Model file for the job. Use its own axes, mm. Face numbers are marked on the shaded views. A direction names the side the tool comes from. Give positions to 0.01 mm unless a question says otherwise; leave off trailing zeros. Write each loop counter-clockwise with the first axis right and the second up, starting at its lowest first coordinate (ties: lowest second). Pieces come first, ordered by that corner, then holes. Notation, with made-up numbers: M 74,46.5 L 90,46.5 A14 ccw 90,65.5 Z; hole C -18.75,63.5 d10. An arc over 180 degrees is marked long. Answer as a JSON object with one key per item and string values. Group by question number.
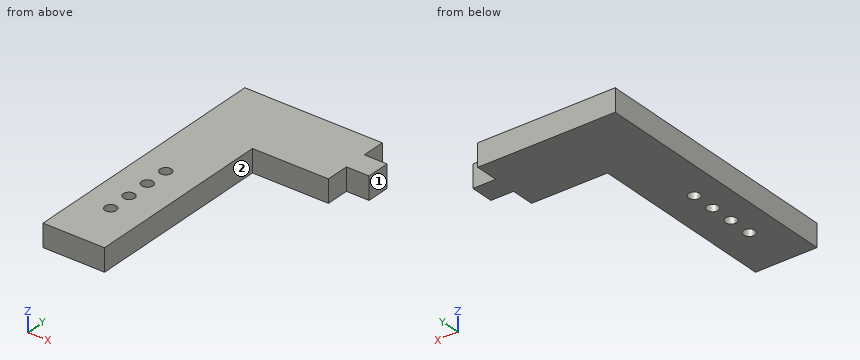
```python
from build123d import *

# Parameters (mm, degrees)
SKETCH1_W           = 13.462
SKETCH1_H           = 57.15
BOSS_EXTRUDE1_DEPTH = 4.9609375
SKETCH2_W           = 4.9609375
SKETCH2_H           = 15.24
BOSS_EXTRUDE2_DEPTH = 21.59
SKETCH5_R           = 1.2446
SKETCH5_R_2         = 1.25
SKETCH5_R_3         = 1.24968
CUT_EXTRUDE2_DEPTH  = 5.9609375
SKETCH6_OUTSIDE_W   = 20.407
SKETCH6_OUTSIDE_H   = 72.596
SKETCH6_OUTSIDE_W_2 = 4.9609375
SKETCH6_OUTSIDE_H_2 = 5.08
CUT_EXTRUDE3_DEPTH  = 4.9609375


with BuildPart() as part:
    # Sketch1 → Boss-Extrude1 (new body)
    with BuildSketch(Plane.XY):
        Rectangle(SKETCH1_W, SKETCH1_H)
    extrude(amount=BOSS_EXTRUDE1_DEPTH)

    # Sketch2 → Boss-Extrude2 (add)
    with BuildSketch(Plane(origin=(6.731, 0, 0), x_dir=(0, 0, -1), z_dir=(1, 0, 0))):
        with Locations((-2.48046875, 20.955)):
            Rectangle(SKETCH2_W, SKETCH2_H)
    extrude(amount=BOSS_EXTRUDE2_DEPTH)

    # Sketch5 → Cut-Extrude2 (cut, through all)
    with BuildSketch(Plane(origin=(0, 0, 0), x_dir=(-1, 0, 0), z_dir=(0, 0, -1))):
        with Locations((0.502153829, -17.4625)):
            Circle(SKETCH5_R)
        with Locations((0.502153829, -12.2625)):
            Circle(SKETCH5_R_2)
        with Locations((0.502153829, -7.0625)):
            Circle(SKETCH5_R_3)
        with Locations((0.502153829, -1.8625)):
            Circle(SKETCH5_R_3)
    extrude(amount=-CUT_EXTRUDE2_DEPTH, mode=Mode.SUBTRACT)

    # Sketch6 outside → Cut-Extrude3 (cut)
    with BuildSketch(Plane(origin=(28.321, 0, 0), x_dir=(0, 0, -1), z_dir=(1, 0, 0))):
        with Locations((-2.4805, 0)):
            Rectangle(SKETCH6_OUTSIDE_W, SKETCH6_OUTSIDE_H)
        with Locations((-2.48046875, 20.955)):
            Rectangle(SKETCH6_OUTSIDE_W_2, SKETCH6_OUTSIDE_H_2, mode=Mode.SUBTRACT)
    extrude(amount=-CUT_EXTRUDE3_DEPTH, mode=Mode.SUBTRACT)


solid = part.part
```
Q1. Drop flat-ended pins along their axis: P1, Ø1.5, axis at x = 25, z = 1.5, coming from the +Y side (3 decimals); P2, Ø2.5, axis at y = 15, z = 3, coming from the +X side; P3, Ø2.5, axis at y = -14, z = 3.5, coming from the +X side. Give the stop position or say it passes through.
Q2. Slice it at B-B, the plane x = 26.5. Write the cut outline in (y, z) (3 decimals).
Q3. Wall check: L1, parallel to Y at x = -1, z = 0.55 (3 decimals); L2, parallel to Y at x = 7, z = 1.65 (3 decimals); L3, parallel to X at y = -25, z = 4.4. Give the ranges that are in metal, low to high.
Q4. Slice it at C-C, the plane y = -15. Write the cut outline in (x, z).
Q5. 3-axis set-ups, long thin cutter, end or side, ignore diameter. For the marked faces 1 and 2: which of +Z, -Z, +X, -X, +Y, -Y reach the whole face in a straight line?
Q6. Slice it at A-A, the plane z = 2.95. Count the separate pieces of the cut face and the enclosed holes in it, then the cut area to 3 significant figures.
Solved:
{
 "1": {"P1": "stops at y = 23.495", "P2": "stops at x = 23.36", "P3": "stops at x = 6.73"},
 "2": {"outline": "M 18.415,0 L 23.495,0 L 23.495,4.961 L 18.415,4.961 Z"},
 "3": {"L1": "y = -28.575 to -18.603, -16.322 to -13.409, -11.116 to -8.209, -5.916 to -3.009, -0.716 to 28.575", "L2": "y = 13.335 to 28.575", "L3": "x = -6.73 to 6.73"},
 "4": {"outline": "M -6.73,0 L 6.73,0 L 6.73,4.96 L -6.73,4.96 Z"},
 "5": {"face 1": "+Z, -Z, +X, +Y, -Y", "face 2": "+Z, -Z, +X, -Y"},
 "6": {"separate pieces": "1", "enclosed holes": "4", "area": "1,030 mm²"}
}
